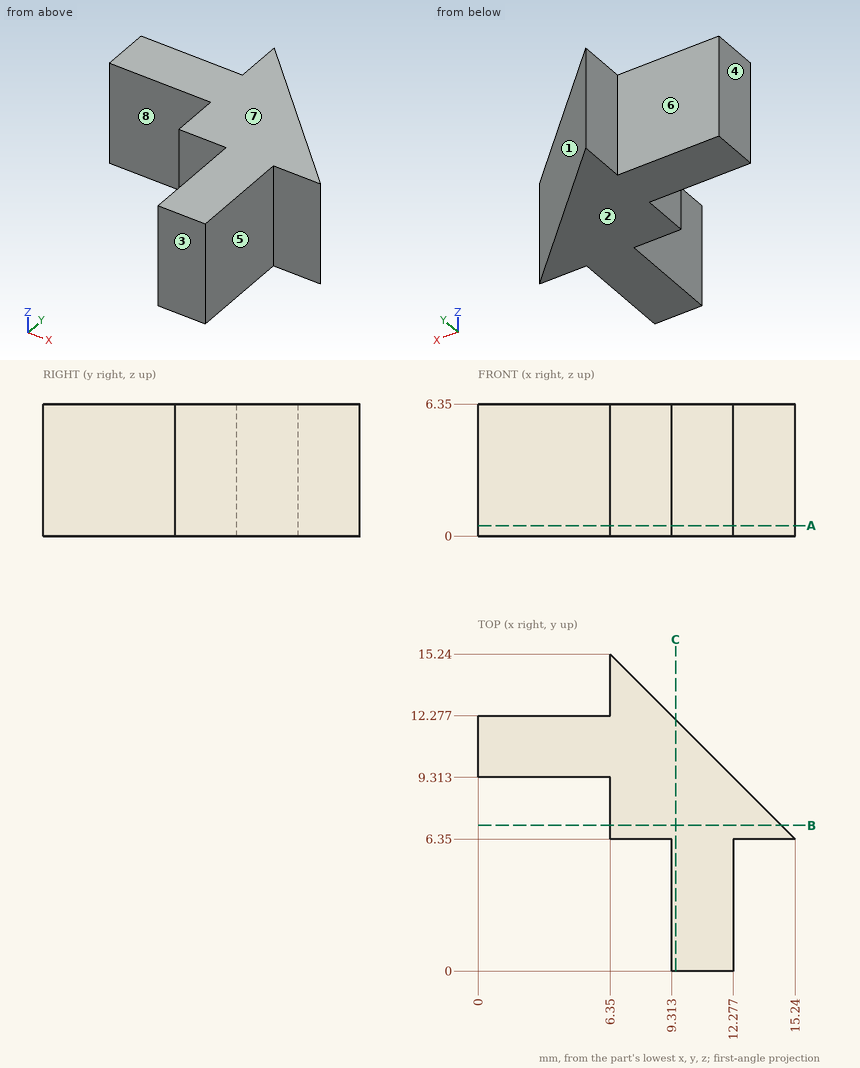
Verification items for this drawing (mm, ordinates from the low corner). A direction names the side the tool comes from. Coordinates: 2 decimals unless noted, no trailing zeros. Write each loop counter-clockwise with the first axis right and the second up, starting at its lowest first coordinate (ties: lowest second). Pieces come first, ordered by that corner, then holes. Notation, with made-up numbers: (77, 68) - (87, 68) arc R16 cw to (87, 93) - close; hole circle Ø11 at (-12, 57). An arc over 180 degrees is marked (long way). One line per question, with ' | ' between items.
Item 1: Access from +Z, -Z, +X, -X, +Y, -Y to the whole of each face (thin tool, end or side, straight path). Record for the marked faces 4, 5, 6, 7 and 8.
Determined:
face 4: +Z, -Z, -X, +Y, -Y | face 5: +Z, -Z, +X, -Y | face 6: +Z, -Z, -X, +Y | face 7: +Z, +X, -X, +Y, -Y | face 8: +Z, -Z, -X, -Y
Item 2: Thickness scan on line 1 (X direction, y = 4.75, z = 3); line 2 (X direction, y = 13.75, z = 1.25). Record the ranges inside material, lowest first. Write a range as [from, to].
Determined:
line 1: x = [9.31, 12.28] | line 2: x = [6.35, 7.84]
Item 3: Sectioned sample at C-C on x = 9.5. Record the boundary of the cut face in (y, z).
Determined:
outline: (0, 0) - (12.09, 0) - (12.09, 6.35) - (0, 6.35) - close
Item 4: Mould release check, pull along Y, two halves, no side actions. Record for the marked faces 1, 2 and 3: pulls with the +Y half, pulls with the -Y half, needs draft (parallel to the pull), parting line crosses it, or undercut.
Determined:
face 1: pulls with the +Y half | face 2: needs draft | face 3: pulls with the -Y half
Item 5: Sectioned sample at B-B on y = 7. Record the boundary of the cut face in (x, z).
Determined:
outline: (6.35, 0) - (14.59, 0) - (14.59, 6.35) - (6.35, 6.35) - close
Item 6: Gauge pin test, flat ends, axial feed: P1, Ø1.9, axis at y = 2, z = 2.5, coming from the -X side; P2, Ø3, axis at x = 4.5, z = 3, coming from the +Y side; P3, Ø0.9, axis at y = 8, z = 3, coming from the -X side. Record the tip position at first contact, or that the pin passes through.
Determined:
P1: stops at x = 9.31 | P2: stops at y = 12.28 | P3: stops at x = 6.35
Item 7: Sectioned sample at A-A on z = 0.5. Record the boundary of the cut face in (x, y).
Determined:
outline: (0, 9.31) - (6.35, 9.31) - (6.35, 6.35) - (9.31, 6.35) - (9.31, 0) - (12.28, 0) - (12.28, 6.35) - (15.24, 6.35) - (6.35, 15.24) - (6.35, 12.28) - (0, 12.28) - close
